CAD build for the part. Positions are in the model's coordinates, mm. A direction names the side the tool comes from. Give positions to 0.01 mm unless a question says otherwise; leave off trailing zeros. Write each loop counter-clockwise with the first axis right and the second up, starting at its lowest first coordinate (ties: lowest second). Pieces come first, ordered by that corner, then holes. Notation, with made-up numbers: (67, 57.5) - (99, 57.5) arc R13 ccw to (99, 68.5) - close; hole circle Ø2 at (-22.75, -4.75). An arc over 180 degrees is marked (long way). Write item = value, one per line. Start each with the question number.
```python
from build123d import *

# Parameters (mm, degrees)
EXTRUDE_1_DEPTH     = 50
SKETCH_5_R          = 17.5
CUT_EXTRUDE_1_DEPTH = 51


with BuildPart() as part:
    # 草圖1 → 填料-伸長1 (new body)
    with BuildSketch(Plane(origin=(0, 0, 0), x_dir=(1, 0, 0), z_dir=(0, 1, 0))):
        with BuildLine():
            Line((-120, 100), (-60, 100))
            ThreePointArc((-60, 100), (-17.573593129, 82.426406871), (0, 40))
            Line((0, 40), (0, -40))
            ThreePointArc((0, -40), (-17.573593129, -82.426406871), (-60, -100))
            Line((-60, -100), (-120, -100))
            Line((-120, -100), (-120, -50))
            Line((-120, -50), (-70, 0))
            Line((-70, 0), (-120, 50))
            Line((-120, 50), (-120, 100))
        make_face()
        with BuildLine():
            Line((-64.393398282, 70.606601718), (-32.573593129, 38.786796564))
            ThreePointArc((-32.573593129, 38.786796564), (-32.573593129, 17.573593129), (-53.786796564, 17.573593129))
            Line((-53.786796564, 17.573593129), (-85.606601718, 49.393398282))
            ThreePointArc((-85.606601718, 49.393398282), (-85.606601718, 70.606601718), (-64.393398282, 70.606601718))
        make_face(mode=Mode.SUBTRACT)
        with BuildLine():
            Line((-64.393398282, -70.606601718), (-32.573593129, -38.786796564))
            ThreePointArc((-32.573593129, -38.786796564), (-32.573593129, -17.573593129), (-53.786796564, -17.573593129))
            Line((-53.786796564, -17.573593129), (-85.606601718, -49.393398282))
            ThreePointArc((-85.606601718, -49.393398282), (-85.606601718, -70.606601718), (-64.393398282, -70.606601718))
        make_face(mode=Mode.SUBTRACT)
    extrude(amount=EXTRUDE_1_DEPTH)

    # 掃出1: sweep along a path in 草圖2
    with BuildLine(Plane.XY) as sweep_1_path:
        Line((0, 50), (60, 50))
        ThreePointArc((60, 50), (100.613846605, 41.381154862), (134.226804124, 17.010309278))
        Line((134.226804124, 17.010309278), (197.886597938, -53.505154639))
        ThreePointArc((197.886597938, -53.505154639), (214.693076697, -65.690577431), (235, -70))
        Line((235, -70), (350, -70))
    # 草圖3 → 掃出1 (sweep)
    with BuildSketch(Plane(origin=(0, 0, 0), x_dir=(0, 0, -1), z_dir=(1, 0, 0))):
        Polygon((17.5, 50), (-17.5, 50), (-17.5, 40), (-5, 40), (-5, 10), (-17.5, 10), (-17.5, 0), (17.5, 0), (17.5, 10), (5, 10), (5, 40), (17.5, 40), align=None)
    sweep(path=sweep_1_path.line)

    # 草圖4 → 旋轉1 (revolve)
    with BuildSketch(Plane.XY):
        Polygon((350, -70), (390, -70), (390, -80), (375, -80), (375, -110), (390, -110), (390, -120), (350, -120), align=None)
    revolve(axis=Axis((350, -47.23777031, 0), (0, -1, 0)))

    # 草圖5 → 除料-伸長1 (cut, through all)
    with BuildSketch(Plane(origin=(0, -70, 0), x_dir=(1, 0, 0), z_dir=(0, 1, 0))):
        with Locations((350, 0)):
            Circle(SKETCH_5_R)
    extrude(amount=-CUT_EXTRUDE_1_DEPTH, mode=Mode.SUBTRACT)


solid = part.part
```
1. Cut at B-B (x = -75). Give the cut face in (y, z).
2. Cut at C-C (y = 33.5). Give the cut face in (x, z) (3 decimals).
3. Cut at D-D (z = 60). Give the cut face in (x, y).
4. Wall check: line 1 along Z through (x, y) = (350, -108); line 2 along X through (y, z) = (-97, 0); line 3 along X through (y, z) = (41, -53). Give the ranges that are in metal, low to high.
5. Pin check, flat tips, straight feed: pin 1 Ø10 at (y, z) = (-2, -19) entering from +X; pin 2 Ø14 at (x, z) = (19.5, -12.5) entering from -Y; pin 3 Ø8 at (x, y) = (310, -77.5) entering from +Z. Stop position of each tip, or through.
6. Cut at A-A (x = 350). Give the cut face in (y, z), then the cut area to 3 significant figures.
7. Tool access for faces 1 (the flat face through (158, -15, 17.5)), 2 (the flat face through (314, -70, 1)), 3 (the flat face through (136.812, -45.545, 11.163)): list every direction of +Z, -Z, +X, -X, +Y, -Y with a clear straight run to the whole face (end or side of a thin tool).
8. Mould opens along X. For faces 4 (the cylindrical face through (389.97, -75.07, -1.51)), 5 (the cylindrical face through (100.078, 41.617, 0.245)), 6 (the flat face through (30, 40, -11)) say: +X half, -X half, draft (parallel to the pull), parting line (faces both ways), or undercut.
Output:
q1.outline = (0, -100) - (50, -100) - (50, -75) - (0, -75) - close; (0, -38.79) - (50, -38.79) - (50, -5) - (0, -5) - close; (0, 5) - (50, 5) - (50, 38.79) - (0, 38.79) - close; (0, 75) - (50, 75) - (50, 100) - (0, 100) - close
q2.outline = (-120, -100) - (-60, -100) arc R60 ccw to (0, -40) - (0, -5) - (93.582, -5) - (93.582, -17.5) - (115.025, -17.5) - (115.025, 17.5) - (93.582, 17.5) - (93.582, 5) - (0, 5) - (0, 40) arc R60 ccw to (-60, 100) - (-120, 100) - (-120, 50) - (-70, 0) - (-120, -50) - close; hole (-85.607, -49.393) arc R15 ccw to (-64.393, -70.607) - (-32.574, -38.787) arc R15 ccw to (-53.787, -17.574) - close; hole (-85.607, 49.393) - (-53.787, 17.574) arc R15 ccw to (-32.574, 38.787) - (-64.393, 70.607) arc R15 ccw to start
q3.outline = (-120, 0) - (-90, 0) - (-90, 50) - (-120, 50) - close; (-53.79, 0) - (-3.43, 0) - (-3.43, 50) - (-53.79, 50) - close
q4.line_1 = -25 to -17.5, 17.5 to 25
q4.line_2 = 171.2 to 332.5, 367.5 to 375
q4.line_3 = -120 to -88.27, -46.79 to -1.43
q5.pin_1 = 155.69
q5.pin_2 = 0
q5.pin_3 = 17.5
q6.outline = (-120, -40) - (-110, -40) - (-110, -25) - (-80, -25) - (-80, -40) - (-70, -40) - (-70, -17.5) - (-120, -17.5) - close; (-120, 17.5) - (-70, 17.5) - (-70, 40) - (-80, 40) - (-80, 25) - (-110, 25) - (-110, 40) - (-120, 40) - close
q6.area = 1,350 mm2
q7.face_1 = +Z, +Y, -Y
q7.face_2 = +Z, -Z, +X, +Y
q7.face_3 = +Z
q8.face_4 = parting line
q8.face_5 = +X half
q8.face_6 = undercut
